The model under review builds one solid part; all positions refer to its coordinate system, in mm. Face numbers are marked on the shaded views. Coordinates: 2 decimals unless noted, no trailing zeros. Order: outer loops, then holes, each group sorted by start corner. A loop starts at its lowest first (then second) coordinate and runs counter-clockwise, first axis right, second up. Notation, with made-up numbers: M 3.25,31 L 35.25,31 A26 ccw 35.25,68 Z; hole C -3.75,15 d6. An arc over 180 degrees is marked long. Answer in a Markdown table with one row per item.
Autodesk Fusion 360 part; units mm, degrees
sketch "Sketch1" plane through (0, 0, 0) normal (0, 1, 0) x (1, 0, 0)
  line L0 (60.3, -37.35) -> (-60.3, -37.35)
  line L1 (-60.3, -37.35) -> (-60.3, 31.2432)
  line L2 (-60.3, 37.35) -> (60.3, 37.35)
  line L3 (60.3, 37.35) -> (60.3, -37.35)
  line L4 (60.3, -37.35) -> (-60.3, 37.35) construction
  line L5 (-60.3, -37.35) -> (60.3, 37.35) construction
  line L6 (-66.3, 43.35) -> (66.3, 43.35)
  line L7 (66.3, 43.35) -> (66.3, -43.35)
  line L8 (66.3, -43.35) -> (-66.3, -43.35)
  line L9 (-66.3, -43.35) -> (-66.3, 43.35)
  line L10 (-60.3, -37.35) -> (-54.5, -37.35)
  line L11 (-60.3, -31.35) -> (-60.3, -37.35)
  line L12 (60.3, -37.35) -> (54.5, -37.35)
  line L13 (60.3, -31.35) -> (60.3, -37.35)
  line L14 (-60.3, 37.35) -> (-54.5, 37.35)
  line L15 (-60.3, 31.35) -> (-60.3, 37.35)
  line L16 (60.3, 37.35) -> (54.5, 37.35)
  line L17 (60.3, 31.35) -> (60.3, 37.35)
  circle A0 centre (-57.4, -34.35) radius 1
  circle A1 centre (57.4, -34.35) radius 1
  line L18 (2.5, 0) -> (20, 0)
  circle A2 centre (57.4, 34.35) radius 1
  circle A3 centre (-57.4, 34.35) radius 1
  circle A4 centre (0, -40.35) radius 1
  circle A5 centre (0, 40.35) radius 1
  circle A6 centre (57.4, -34.35) radius 4.25
  circle A7 centre (57.4, 34.35) radius 4.25
  circle A8 centre (-57.4, 34.35) radius 4.25
  circle A9 centre (-57.4, -34.35) radius 4.25
  point P0 (-57.4, 34.35)
  dimension "d1" = 120.6
  dimension "d2" = 74.7
  dimension "d6" = 5.8
  dimension "d7" = 6
  dimension "d8" = 5.8
  dimension "d9" = 6
  dimension "d10" = 5.8
  dimension "d11" = 6
  dimension "d12" = 5.8
  dimension "d13" = 6
  dimension "d16" = 2
  dimension "d17" = 2
  dimension "d18" = 2
  dimension "d22" = 2
  dimension "d23" = 8.5
  dimension "d24" = 8.5
  dimension "d25" = 8.5
  dimension "d26" = 8.5
extrude "Extrude1" add sketch "Sketch1" along normal blind 3 contours L0 L3 L12 L13 A6 | L0 L3 L12 L13 A6 | L0 L1 L2 L3 A6 A7 A8 A9 | L0 L1 L10 L11 A9 | L0 L1 L10 L11 A9 | L2 L3 L16 L17 A7 | L2 L3 L16 L17 A7 | A8 | L6 L7 L8 L9 | A0 | A1 | A2 | A3 | A4 | A5
extrude "Extrude3" cut sketch "Sketch1" along normal blind 10 contours A0 | A1 | A2 | A3
extrude "Extrude4" add sketch "Sketch1" against normal blind 6.5 contours L0 L3 L12 L13 A6 | L0 L3 L12 L13 A6 | L0 L1 L10 L11 A9 | L0 L1 L10 L11 A9 | L2 L3 L16 L17 A7 | L2 L3 L16 L17 A7 | A8
sketch "Sketch2" plane through (0, 0, 0) normal (0, 1, 0) x (1, 0, 0)
extrude "Extrude5" cut sketch "Sketch1" along normal blind 10 contours L0 L1 L2 L3 A6 A7 A8 A9
sketch "Sketch3" plane through (0, 3, 0) normal (0, 1, 0) x (-1, 0, 0)
  arc A0 (54.3896, 37.35) -> (60.3, 31.2432) centre (57.4, 34.35) ccw
  line L0 (60.3, 31.2432) -> (60.3, -31.2432)
  arc A1 (60.3, -31.2432) -> (54.3896, -37.35) centre (57.4, -34.35) ccw
  line L1 (54.3896, -37.35) -> (-54.3896, -37.35)
  arc A2 (-54.3896, -37.35) -> (-60.3, -31.2432) centre (-57.4, -34.35) ccw
  line L2 (-60.3, -31.2432) -> (-60.3, 31.2432)
  arc A3 (-60.3, 31.2432) -> (-54.3896, 37.35) centre (-57.4, 34.35) ccw
  line L3 (-54.3896, 37.35) -> (54.3896, 37.35)
  circle A4 centre (57.4, -34.35) radius 1
  circle A5 centre (57.4, 34.35) radius 1
  circle A6 centre (-57.4, -34.35) radius 1
  circle A7 centre (-57.4, 34.35) radius 1
  line L4 (66.3, 43.35) -> (-66.3, 43.35)
  line L5 (-66.3, 43.35) -> (-66.3, -43.35)
  line L6 (-66.3, -43.35) -> (66.3, -43.35)
  line L7 (66.3, -43.35) -> (66.3, 43.35)
  line L8 (-5, -37.35) -> (5, -37.35)
  line L9 (5, -37.35) -> (5, 37.35)
  line L10 (5, 37.35) -> (-5, 37.35)
  line L11 (-5, 37.35) -> (-5, -37.35)
  line L12 (-5, -37.35) -> (5, 37.35) construction
  line L13 (5, -37.35) -> (-5, 37.35) construction
  line L14 (60.3, 5) -> (-60.3, 5)
  line L15 (-60.3, 5) -> (-60.3, -5)
  line L16 (-60.3, -5) -> (60.3, -5)
  line L17 (60.3, -5) -> (60.3, 5)
  line L18 (60.3, 5) -> (-60.3, -5) construction
  line L19 (-60.3, 5) -> (60.3, -5) construction
  dimension "d31" = 10
  dimension "d32" = 10
extrude "Extrude6" add sketch "Sketch3" against normal blind 3 contours L3 L9 L10 L11 L14 | L0 L9 L14 L16 L17 | L9 L11 L14 L16 | L2 L11 L14 L15 L16 | L1 L8 L9 L11 L16
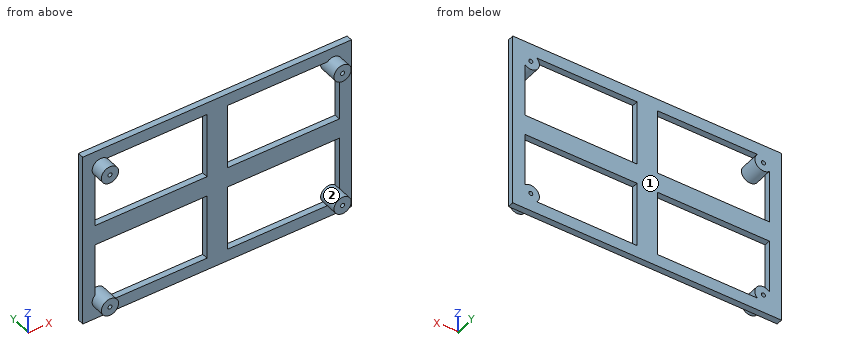
(1) Take a section at A-A (y = -2.75). Write out the cut boundary in (x, z).
Report:
| item | result |
|---|---|
| outline | C -57.4,-34.35 d8.5; C -57.4,34.35 d8.5; C 57.4,-34.35 d8.5; C 57.4,34.35 d8.5; hole C -57.4,-34.35 d2; hole C -57.4,34.35 d2; hole C 57.4,-34.35 d2; hole C 57.4,34.35 d2 |
(2) Take a section at D-D (z = 0). Write out the cut boundary in (x, y).
Report:
| item | result |
|---|---|
| outline | M -66.3,0 L 66.3,0 L 66.3,3 L -66.3,3 Z |
(3) Take a section at C-C (x = -6.5). Write out the cut boundary in (y, z), then the cut area to 3 significant figures.
Report:
| item | result |
|---|---|
| outline | M 0,-43.35 L 3,-43.35 L 3,-37.35 L 0,-37.35 Z; M 0,-5 L 3,-5 L 3,5 L 0,5 Z; M 0,37.35 L 3,37.35 L 3,43.35 L 0,43.35 Z |
| area | 66.0 mm^2 |
(4) The part is to be moulded in two halves that separate along X. For the marked faces 1 and 2, say which applies: +X half, -X half, draft (parallel to the pull), parting line (faces both ways), or undercut.
Report:
| item | result |
|---|---|
| face 1 | draft |
| face 2 | undercut |
(5) To check wall thickness, follow line 1 (Z direction, x = -57.4, y = -1.25); line 2 (Z direction, x = -22.5, y = 2); line 3 (X direction, y = -4.5, z = -34.35). State the ranges of each line that lie inside material, in increasing order. Write a range as [from, to].
Report:
| item | result |
|---|---|
| line 1 | [-38.6, -35.35], [-33.35, -30.1], [30.1, 33.35], [35.35, 38.6] |
| line 2 | [-43.35, -37.35], [-5, 5], [37.35, 43.35] |
| line 3 | [-61.65, -58.4], [-56.4, -53.15], [53.15, 56.4], [58.4, 61.65] |
(6) Take a section at B-B (z = -12). Write out the cut boundary in (x, y).
Report:
| item | result |
|---|---|
| outline | M -66.3,0 L -60.3,0 L -60.3,3 L -66.3,3 Z; M -5,0 L 5,0 L 5,3 L -5,3 Z; M 60.3,0 L 66.3,0 L 66.3,3 L 60.3,3 Z |
